Verification items for the finished model (mm, model axes). A direction names the side the tool comes from. Coordinates: 2 decimals unless noted, no trailing zeros. Write each loop counter-clockwise with the first axis right and the second up, starting at its lowest first coordinate (ties: lowest second). Pieces come first, ordered by that corner, then holes. Notation, with made-up numbers: (22.25, 69) -> (27.25, 69) arc R36 cw to (27.25, 107) -> close; hole circle Ø8 at (22, 22.25). An arc over 180 degrees is marked (long way). Answer in a Markdown table with one row per item.
```python
from build123d import *

# Parameters (mm, degrees)
L_ANGLE_EQUAL_3_6X5_1_DEPTH = 650


with BuildPart() as part:
    # Sketch1 → L angle (equal) 3.6X5(1) (new body)
    with BuildSketch(Plane.YZ):
        with BuildLine():
            Line((36, 0), (0, 0))
            Line((0, 0), (0, -36))
            Line((0, -36), (3.333333333, -36))
            ThreePointArc((3.333333333, -36), (4.511844635, -35.511844635), (5, -34.333333333))
            Line((5, -34.333333333), (5, -9.5))
            ThreePointArc((5, -9.5), (6.318019485, -6.318019485), (9.5, -5))
            Line((9.5, -5), (34.333333333, -5))
            ThreePointArc((34.333333333, -5), (35.511844635, -4.511844635), (36, -3.333333333))
            Line((36, -3.333333333), (36, 0))
        make_face()
    extrude(amount=L_ANGLE_EQUAL_3_6X5_1_DEPTH)


solid = part.part
```
1. Sectioned sample at C-C, the plane y = 26. Record the cut outline in (x, z).
Findings below:
| item | result |
|---|---|
| outline | (0, -5) -> (650, -5) -> (650, 0) -> (0, 0) -> close |
2. Sectioned sample at A-A, the plane x = 77.5. Record the cut outline in (y, z).
Findings below:
| item | result |
|---|---|
| outline | (0, -36) -> (3.33, -36) arc R1.67 ccw to (5, -34.33) -> (5, -9.5) arc R4.5 cw to (9.5, -5) -> (34.33, -5) arc R1.67 ccw to (36, -3.33) -> (36, 0) -> (0, 0) -> close |
3. Material ranges on probe 1 along Y at (x, z) = (386.5, -28); probe 2 along Z at (x, y) = (529, 29.5); probe 3 along Z at (x, y) = (447.5, 3.5), recorded low to high. Write a range as from..to.
Findings below:
| item | result |
|---|---|
| probe 1 | y = 0..5 |
| probe 2 | z = -5..0 |
| probe 3 | z = -35.99..0 |
4. Go/stop test with flat-tipped pins: pin 1 (8 mm diameter, centred on x = 563, y = 17, fed in from -Z); pin 2 (12.5 mm diameter, centred on x = 284, z = -18, fed in from +Y); pin 3 (6 mm diameter, centred on x = 238, y = 10.5, fed in from -Z). Record where each tip stops, or that it passes through.
Findings below:
| item | result |
|---|---|
| pin 1 | stops at z = -5 |
| pin 2 | stops at y = 5 |
| pin 3 | stops at z = -5.47 |
5. Access from +Z, -Z, +X, -X, +Y, -Y to the whole of each face (thin tool, end or side, straight path). Record for faces 1 (the face through (650, 11.2, -4.6)), 2 (the face through (320, 22, -5)).
Findings below:
| item | result |
|---|---|
| face 1 | +Z, -Z, +X, +Y, -Y |
| face 2 | -Z, +X, -X, +Y |
6. Sectioned sample at B-B, the plane z = -17.5. Record the cut outline in (x, y).
Findings below:
| item | result |
|---|---|
| outline | (0, 0) -> (650, 0) -> (650, 5) -> (0, 5) -> close |
